```python
from build123d import *

# Parameters (mm, degrees)
F1_DEPTH = 63.5
F0_W     = 25.4
F0_H     = 19.05
F2_DEPTH = 25.4
F3_DEPTH = 12.7
F5_R     = 5.08
F6_R     = 11.3614366128
F7_DEPTH = 28.575


with BuildPart() as f1:
    # F0 (on Front) → F1 (new body, symmetric)
    with BuildSketch(Plane.XZ):
        Polygon((-41.275, -9.525), (41.275, -9.525), (41.275, 9.525), (22.225, 9.525), (-41.275, 9.525), align=None)
    extrude(amount=F1_DEPTH, both=True)

    # F0 (on Front) → F2 (join, symmetric)
    with BuildSketch(Plane.XZ):
        with BuildLine():
            Line((22.225, 9.525), (41.275, 9.525))
            Line((41.275, 9.525), (41.275, 27.0002))
            ThreePointArc((41.275, 27.0002), (45.9246798487, 38.2255201513), (57.15, 42.8752))
            Line((57.15, 42.8752), (60.325, 42.8752))
            Line((60.325, 42.8752), (60.325, 61.9252))
            Line((60.325, 61.9252), (57.15, 61.9252))
            ThreePointArc((57.15, 61.9252), (32.4542956671, 51.6959043329), (22.225, 27.0002))
            Line((22.225, 27.0002), (22.225, 9.525))
        make_face()
        with Locations((73.025, 52.4002)):
            Rectangle(F0_W, F0_H)
    extrude(amount=F2_DEPTH, both=True)

    # F0 (on Front) → F3 (join, symmetric)
    with BuildSketch(Plane.XZ):
        with BuildLine():
            add(Edge.make_bspline(
                [(-41.275, 9.525), (-40.521685034, 43.8802801073), (5.2034435794, 62.1158964932), (57.15, 61.9252)],
                knots=[0, 0, 0, 0, 111.5045361635, 111.5045361635, 111.5045361635, 111.5045361635], degree=3))
            Line((-41.275, 9.525), (22.225, 9.525))
            Line((22.225, 9.525), (22.225, 27.0002))
            ThreePointArc((22.225, 27.0002), (32.4542956671, 51.6959043329), (57.15, 61.9252))
        make_face()
    extrude(amount=F3_DEPTH, both=True)

    # F0 (on Front) → F4 (revolve)
    with BuildSketch(Plane.XZ):
        Polygon((85.725, 66.675), (85.725, 61.9252), (85.725, 42.8752), (85.725, 38.1), (111.125, 38.1), (111.125, 66.675), align=None)
    revolve(axis=Axis((85.725, 0, 52.3875), (0, 0, 1)))

    # F5
    f5_edges = [f1.edges().sort_by_distance(p)[0] for p in [
        (41.275, -63.5, 0),
        (-41.275, -63.5, 0),
        (-41.275, 63.5, 0),
        (41.275, 63.5, 0),
    ]]
    fillet(f5_edges, radius=F5_R)

    # F6 (on face) → F7 (cut)
    with BuildSketch(Plane.XY.offset(66.675)):
        with Locations((85.725, 0)):
            Circle(F6_R)
    extrude(amount=-F7_DEPTH, mode=Mode.SUBTRACT)


solid = f1.part
```
Verification items for the finished model (mm, model axes). A direction names the side the tool comes from. Coordinates: 2 decimals unless noted, no trailing zeros. Loops run counter-clockwise (first coordinate to the right, second up) from the corner with the lowest first, then second, coordinate; pieces in that order, holes last. Notation, with made-up numbers: (14, 10.5) -> (51, 10.5) arc R25 cw to (51, 42.5) -> close; hole circle Ø10 at (31, -7.5). An arc over 180 degrees is marked (long way). Answer in a Markdown table with one row per item. Add a question column.
1. Material ranges on probe 1 along Y at (x, z) = (10.5, 43); probe 2 along X at (y, z) = (48.5, 5) (3 decimals); probe 3 along Z at (x, y) = (7, 52.5) (3 decimals), recorded low to high. Write a range as [from, to].
2. Section check A-A, the plane y = 39.5. Enter the section's corners in (x, z) (3 decimals), then the cut area to 3 significant figures.
3. Draft check along X on faces 4 (the face through (45.8, -0.4, 38.1)), 5 (the face through (-2, 12.7, 30)), 6 (the face through (-39.8, 62, -0.1)). Enter one of: +X half, -X half, draft (parallel to the pull), parting line (faces both ways), or undercut.
4. Depth check by flat-ended pin: P1, Ø8.5, axis at x = 72.5, y = 11.5, coming from the -Z side; P2, Ø4, axis at x = -18.5, y = 16, coming from the +Z side (3 decimals); P3, Ø12, axis at x = 35, y = -22.5, coming from the +Z side. Enter the tip coordinate at first touch or a pass-through.
5. Access from +Z, -Z, +X, -X, +Y, -Y to the whole of each face (thin tool, end or side, straight path). Record for faces 1 (the face through (60, 2, 42.875)), 2 (the face through (75, -5, 38.1)), 3 (the face through (-2, -12.7, 30)).
Derived:
| question | item | result |
|---|---|---|
| 1 | probe 1 | y = [-12.7, 12.7] |
| 1 | probe 2 | x = [-41.275, 41.275] |
| 1 | probe 3 | z = [-9.525, 9.525] |
| 2 | outline | (-41.275, -9.525) -> (41.275, -9.525) -> (41.275, 9.525) -> (-41.275, 9.525) -> close |
| 2 | area | 1,570 mm² |
| 3 | face 4 | undercut |
| 3 | face 5 | draft |
| 3 | face 6 | -X half |
| 4 | P1 | stops at z = 38.1 |
| 4 | P2 | stops at z = 9.525 |
| 4 | P3 | stops at z = 57.97 |
| 5 | face 1 | -Z |
| 5 | face 2 | -Z, +X, +Y, -Y |
| 5 | face 3 | +Z, -X, -Y |
